Design review of the part built by this model. Coordinates are the model's own, in mm. A direction names the side the tool comes from. Round coordinates to 2 decimals unless told otherwise and drop trailing zeros. Write each loop counter-clockwise with the first axis right and the second up, starting at its lowest first coordinate (ties: lowest second). Pieces come first, ordered by that corner, then holes. Notation, with made-up numbers: (8.25, -32) - (28.25, -32) arc R27 cw to (28.25, 4) - close; hole circle Ø11 at (-38, 41). An arc over 180 degrees is marked (long way). Use one line per item in the form item = value.
```python
from build123d import *

# Parameters (mm, degrees)
SKETCH1_R             = 3.25
BOSS_EXTRUDE1_DEPTH   = 1.75
CUT_EXTRUDE1_DEPTH    = 0.95
F_2_CLEARANCE_HOLE1_D = 2.4384


with BuildPart() as part:
    # Sketch1 → Boss-Extrude1 (new, symmetric)
    with BuildSketch(Plane(origin=(0, 0, 0), x_dir=(1, 0, 0), z_dir=(0, 1, 0))):
        with Locations(Location((0, 0, 0), (0, 0, 270))):
            Circle(SKETCH1_R)
    extrude(amount=BOSS_EXTRUDE1_DEPTH, both=True)

    # Sketch2 → Cut-Extrude1 (cut, symmetric)
    with BuildSketch(Plane(origin=(0, 0, 0), x_dir=(1, 0, 0), z_dir=(0, 1, 0))):
        Polygon((2.829016319, 0), (1.41450816, 2.45), (-1.41450816, 2.45), (-2.829016319, 0), (-1.41450816, -2.45), (1.41450816, -2.45), align=None)
    extrude(amount=CUT_EXTRUDE1_DEPTH, both=True, mode=Mode.SUBTRACT)

    # #2 Clearance Hole1 (through all)
    with Locations(Plane(origin=(0, 1.75, 0), x_dir=(1, 0, 0), z_dir=(0, 1, 0))):
        with Locations((0, 0)):
            Hole(F_2_CLEARANCE_HOLE1_D / 2)


solid = part.part
```
Q1. We need section C-C on y = -0.4. Write out the cut boundary in (x, z), then the cut area to 3 significant figures.
Calculated:
outline = circle Ø6.5 at (0, 0); hole (-2.83, 0) - (-1.41, -2.45) - (1.41, -2.45) - (2.83, 0) - (1.41, 2.45) - (-1.41, 2.45) - close
area = 12.4 mm2
Q2. Draft analysis for pull direction Y (two halves, no side actions). For faces 1 (the flat face through (0, -1.75, 1.4)), 2 (the flat face through (0, 1.75, 1.4)), 3 (the flat face through (2.13, 0.01, -1.21)), 4 (the flat face through (2.112, 0.013, 1.242)), state which applies: released by +Y, released by -Y, zero draft, split by the parting line, or undercut.
Calculated:
face_1 = released by -Y
face_2 = released by +Y
face_3 = undercut
face_4 = undercut
Q3. Machinability: for faces 5 (the cylindrical face through (-1.16, -1.36, -0.37)), 6 (the flat face through (1, -0.95, -1)), which of the approach directions +Z, -Z, +X, -X, +Y, -Y give a long, thin tool a straight path to every point of the face, cutting with its end or side? Answer none if there is none.
Calculated:
face_5 = +Y, -Y
face_6 = none
Q4. We need section A-A on x = 0. Write out the cut boundary in (y, z), then the cut area to 3 significant figures.
Calculated:
outline = (-1.75, -3.25) - (1.75, -3.25) - (1.75, -1.22) - (0.95, -1.22) - (0.95, -2.45) - (-0.95, -2.45) - (-0.95, -1.22) - (-1.75, -1.22) - close; (-1.75, 1.22) - (-0.95, 1.22) - (-0.95, 2.45) - (0.95, 2.45) - (0.95, 1.22) - (1.75, 1.22) - (1.75, 3.25) - (-1.75, 3.25) - close
area = 9.54 mm2
Q5. To check wall thickness, follow line 1 along Y through (x, z) = (-1.5, -1); line 2 along X through (y, z) = (0.8, -2.25); line 3 along X through (y, z) = (1.4, 0.75). State the ranges of each line that lie inside material, in increasing order. Write a range as from..to.
Calculated:
line_1 = -1.75..-0.95, 0.95..1.75
line_2 = -2.35..-1.53, 1.53..2.35
line_3 = -3.16..-0.96, 0.96..3.16
Q6. We need section B-B on z = 0.25. Write out the cut boundary in (x, y), then the cut area to 3 significant figures.
Calculated:
outline = (-3.24, -1.75) - (-1.19, -1.75) - (-1.19, -0.95) - (-2.68, -0.95) - (-2.68, 0.95) - (-1.19, 0.95) - (-1.19, 1.75) - (-3.24, 1.75) - close; (1.19, -1.75) - (3.24, -1.75) - (3.24, 1.75) - (1.19, 1.75) - (1.19, 0.95) - (2.68, 0.95) - (2.68, -0.95) - (1.19, -0.95) - close
area = 8.66 mm2
Q7. We need section D-D on z = 1.75. Write out the cut boundary in (x, y).
Calculated:
outline = (-2.74, -1.75) - (2.74, -1.75) - (2.74, 1.75) - (-2.74, 1.75) - close; hole (-1.82, -0.95) - (1.82, -0.95) - (1.82, 0.95) - (-1.82, 0.95) - close
